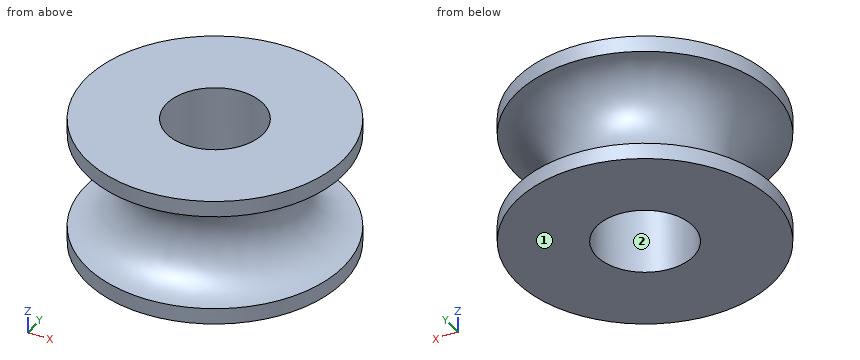
```python
from build123d import *

# Parameters (mm, degrees)
SKETCH1_R           = 25.4
BOSS_EXTRUDE1_DEPTH = 25.4
SKETCH3_R           = 9.525
CUT_EXTRUDE1_DEPTH  = 25.4


with BuildPart() as part:
    # Sketch1 → Boss-Extrude1 (new body)
    with BuildSketch(Plane.XY):
        Circle(SKETCH1_R)
    extrude(amount=BOSS_EXTRUDE1_DEPTH)

    # Sketch2 → Cut-Revolve1 (revolve, cut)
    with BuildSketch(Plane(origin=(0, 0, 0), x_dir=(1, 0, 0), z_dir=(0, 1, 0))):
        with BuildLine():
            Line((25.4, -22.225), (25.4, -3.175))
            ThreePointArc((25.4, -3.175), (15.875, -12.7), (25.4, -22.225))
        make_face()
    revolve(axis=Axis((0, 0, 32.071065699), (0, 0, -1)), mode=Mode.SUBTRACT)

    # Sketch3 → Cut-Extrude1 (cut)
    with BuildSketch(Plane(origin=(0, 0, 0), x_dir=(-1, 0, 0), z_dir=(0, 0, -1))):
        Circle(SKETCH3_R)
    extrude(amount=-CUT_EXTRUDE1_DEPTH, mode=Mode.SUBTRACT)


solid = part.part
```
The listing builds one solid part. Answer for the finished solid, in the listing's coordinates (mm). Face numbers are marked on the shaded views. Round coordinates to 2 decimals unless told otherwise and drop trailing zeros. Order: outer loops, then holes, each group sorted by start corner. A loop starts at its lowest first (then second) coordinate and runs counter-clockwise, first axis right, second up. Notation, with made-up numbers: (57, -14.75) - (95, -14.75) arc R15 ccw to (95, -7.75) - close; hole circle Ø4 at (-1, 34.5). An arc over 180 degrees is marked (long way). Put each result on its own line as item: value. Start each with the question number.
(1) Find section C-C (z = 23.25). Give the vertices of the cut face in (x, y) (3 decimals).
(2) Find section A-A (y = 0). Give the vertices of the cut face in (x, z) (3 decimals).
(3) Find section D-D (z = 10.5). Give the vertices of the cut face in (x, y) (3 decimals).
(4) Determine the mould class of the marked faces 1 and 2 for opening direction X: released by +X, released by -X, zero draft, split by the parting line, or undercut.
(5) Straight lines are drawn through the part: probe 1 along Z at (x, y) = (19.5, 15.5); probe 2 along Z at (x, y) = (14, 14.5); probe 3 along Y at (x, z) = (0, 20) (3 decimals). For each, find the intervals that lie inside material, in ascending order. Write a range as from..to.
(6) Given P1, Ø10, axis at x = -6.5, z = 15, coming from the -Y side; P2, Ø15, axis at x = 0, y = 0, coming from the -Z side; P3, Ø1.5, axis at y = -1.5, z = 12, coming from the -X side; P4, Ø2, axis at y = 15, z = 12.5, coming from the +X side, each flat-ended and moving along its own axis, determine where each tip first touches the part or whether it passes through.
Reply:
1. outline: circle Ø50.8 at (0, 0); hole circle Ø19.05 at (0, 0)
2. outline: (-25.4, 0) - (-9.525, 0) - (-9.525, 25.4) - (-25.4, 25.4) - (-25.4, 22.225) arc R9.525 cw to (-25.4, 3.175) - close; (9.525, 0) - (25.4, 0) - (25.4, 3.175) arc R9.525 cw to (25.4, 22.225) - (25.4, 25.4) - (9.525, 25.4) - close
3. outline: circle Ø32.265 at (0, 0); hole circle Ø19.05 at (0, 0)
4. face 1: zero draft
4. face 2: undercut
5. probe 1: 0..3.19, 22.21..25.4
5. probe 2: 0..4.75, 20.65..25.4
5. probe 3: -19.282..-9.525, 9.525..19.282
6. P1: y = -18.36
6. P2: through
6. P3: x = -15.93
6. P4: x = 7.49
